```python
from build123d import *

# Parameters (mm, degrees)
CROQUIS1_W              = 35
CROQUIS1_H              = 40
CROQUIS1_R              = 1.5
SALIENTE_EXTRUIR1_DEPTH = 3
CROQUIS2_R              = 5
SALIENTE_EXTRUIR2_DEPTH = 40
CROQUIS3_W              = 27
CROQUIS3_H              = 30
CORTAR_EXTRUIR1_DEPTH   = 21.5
CROQUIS4_R              = 5
CROQUIS4_R_2            = 4
SALIENTE_EXTRUIR3_DEPTH = 1
CROQUIS5_R              = 5
CROQUIS5_R_2            = 4
SALIENTE_EXTRUIR4_DEPTH = 1


with BuildPart() as part:
    # Croquis1 → Saliente-Extruir1 (new body)
    with BuildSketch(Plane(origin=(0, 0, 0), x_dir=(1, 0, 0), z_dir=(0, 1, 0))):
        with Locations((17.5, 20)):
            Rectangle(CROQUIS1_W, CROQUIS1_H)
        with Locations((2.5, 35)):
            Circle(CROQUIS1_R, mode=Mode.SUBTRACT)
        with Locations((32.5, 35)):
            Circle(CROQUIS1_R, mode=Mode.SUBTRACT)
        with Locations((32.5, 5)):
            Circle(CROQUIS1_R, mode=Mode.SUBTRACT)
        with Locations((2.5, 5)):
            Circle(CROQUIS1_R, mode=Mode.SUBTRACT)
    extrude(amount=SALIENTE_EXTRUIR1_DEPTH)

    # Croquis2 → Saliente-Extruir2 (add)
    with BuildSketch(Plane.XY):
        with BuildLine():
            Line((24.5, 16.5), (24.5, 6.880942837))
            ThreePointArc((24.5, 6.880942837), (25.636701839, 4.136701839), (28.380942837, 3))
            Line((28.380942837, 3), (6.5, 3))
            ThreePointArc((6.5, 3), (9.328427125, 4.171572875), (10.5, 7))
            Line((10.5, 7), (10.5, 16.5))
            ThreePointArc((10.5, 16.5), (17.5, 23.5), (24.5, 16.5))
        make_face()
        with Locations((17.5, 16.5)):
            Circle(CROQUIS2_R, mode=Mode.SUBTRACT)
    extrude(amount=-SALIENTE_EXTRUIR2_DEPTH)

    # Croquis3 → Cortar-Extruir1 (cut, through all)
    with BuildSketch(Plane(origin=(0, 3, 0), x_dir=(1, 0, 0), z_dir=(0, 1, 0))):
        with Locations((17.5, 20)):
            Rectangle(CROQUIS3_W, CROQUIS3_H)
    extrude(amount=CORTAR_EXTRUIR1_DEPTH, mode=Mode.SUBTRACT)

    # Croquis4 → Saliente-Extruir3 (add)
    with BuildSketch(Plane.XY.offset(-35)):
        with Locations((17.5, 16.5)):
            Circle(CROQUIS4_R)
        with Locations((17.5, 16.5)):
            Circle(CROQUIS4_R_2, mode=Mode.SUBTRACT)
    extrude(amount=-SALIENTE_EXTRUIR3_DEPTH)

    # Croquis5 → Saliente-Extruir4 (add)
    with BuildSketch(Plane(origin=(0, 0, -5), x_dir=(-1, 0, 0), z_dir=(0, 0, -1))):
        with Locations((-17.5, 16.5)):
            Circle(CROQUIS5_R)
        with Locations((-17.5, 16.5)):
            Circle(CROQUIS5_R_2, mode=Mode.SUBTRACT)
    extrude(amount=-SALIENTE_EXTRUIR4_DEPTH)


solid = part.part
```
The listing builds one solid part. Answer for the finished solid, in the listing's coordinates (mm). A direction names the side the tool comes from. Coordinates: 2 decimals unless noted, no trailing zeros. Loops run counter-clockwise (first coordinate to the right, second up) from the corner with the lowest first, then second, coordinate; pieces in that order, holes last. Notation, with made-up numbers: M 29.5,-29 L 34.5,-29 A21 cw 34.5,5 Z; hole C 57,8.25 d8. An arc over 180 degrees is marked long. Answer as CSV lines item,"result". Start each with the question number.
(1) Find the intervals of material crossed by L1, parallel to Z at x = 2.5, y = 1.1; L2, parallel to X at y = 1.4, z = -5; L3, parallel to Y at x = 17.5, z = -38.55, in increasing order. Write a range as [from, to].
(2) Given pin 1 (4 mm diameter, centred on y = 12, z = -38, fed in from -X); pin 2 (3 mm diameter, centred on x = 20, z = -22, fed in from +Y); pin 3 (1 mm diameter, centred on y = 10, z = -35.5, fed in from +X), each flat-ended and moving along its own axis, determine where each tip first touches the part or whether it passes through.
(3) For faces 4 (the flat face through (10.5, 12, -37)), 5 (the cylindrical face through (16.42, 11.62, -37.97)), 6 (the flat face through (17, 11, -35)), determine the directions among +Z, -Z, +X, -X, +Y, -Y from which every point of the face is accessible in a straight line to the end or side of a thin tool.
(4) The part is cut by section C-C (y = 13). Give the vertices of the cut face in (x, z).
(5) The mould has two halves that part along X. Classify faces 1 (the cylindrical face through (25.607, 4.167, -2.465)), 2 (the flat face through (18, 11, -5)), 3 (the flat face through (15, 20, -36)): pulls with the +X half, pulls with the -X half, needs draft (parallel to the pull), parting line crosses it, or undercut.
(6) The part is cut by section A-A (x = 2.5). Give the vertices of the cut face in (y, z), and give its area (3 significant figures).
(7) The part is cut by section D-D (x = 17.5). Give the vertices of the cut face in (y, z).
(8) The part is cut by section B-B (z = -4.5). Give the vertices of the cut face in (x, y), and give its area (3 significant figures).
Determined:
1,L1,"[-40, -36.5], [-33.5, -6.5], [-3.5, 0]"
1,L2,"[0, 1], [4, 31], [34, 35]"
1,L3,"[0, 11.5], [21.5, 23.5]"
2,pin 1,"x = 10.5"
2,pin 2,"y = 3"
2,pin 3,"x = 24.5"
3,face 4,"+Z, -Z, -X, +Y"
3,face 5,"-Z"
3,face 6,"+X, -X, +Y"
4,outline,"M 10.5,-40 L 13.93,-40 L 13.93,-36 L 15.56,-36 L 15.56,-35 L 10.5,-35 Z; M 10.5,-5 L 15.56,-5 L 15.56,-4 L 13.93,-4 L 13.93,0 L 10.5,0 Z; M 19.44,-36 L 21.07,-36 L 21.07,-40 L 24.5,-40 L 24.5,-35 L 19.44,-35 Z; M 19.44,-5 L 24.5,-5 L 24.5,0 L 21.07,0 L 21.07,-4 L 19.44,-4 Z"
5,face 1,"pulls with the +X half"
5,face 2,"needs draft"
5,face 3,"undercut"
6,outline,"M 0,-40 L 3,-40 L 3,-36.5 L 0,-36.5 Z; M 0,-33.5 L 3,-33.5 L 3,-6.5 L 0,-6.5 Z; M 0,-3.5 L 3,-3.5 L 3,0 L 0,0 Z"
6,area,"102 mm2"
7,outline,"M 0,-40 L 11.5,-40 L 11.5,-36 L 12.5,-36 L 12.5,-35 L 3,-35 L 3,-5 L 12.5,-5 L 12.5,-4 L 11.5,-4 L 11.5,0 L 0,0 Z; M 20.5,-36 L 21.5,-36 L 21.5,-40 L 23.5,-40 L 23.5,-35 L 20.5,-35 Z; M 20.5,-5 L 23.5,-5 L 23.5,0 L 21.5,0 L 21.5,-4 L 20.5,-4 Z"
8,outline,"M 0,0 L 1.09,0 L 1.09,3 L 0,3 Z; M 3.91,0 L 31.09,0 L 31.09,3 L 28.38,3 A3.88 cw 24.5,6.88 L 24.5,16.5 A7 ccw 10.5,16.5 L 10.5,7 A4 cw 6.5,3 L 3.91,3 Z; M 33.91,0 L 35,0 L 35,3 L 33.91,3 Z; hole C 17.5,16.5 d8"
8,area,"310 mm2"
